Verification items for the finished model (mm, model axes). Face numbers are marked on the shaded views. A direction names the side the tool comes from. Give positions to 0.01 mm unless a question says otherwise; leave off trailing zeros. Write each loop counter-clockwise with the first axis right and the second up, starting at its lowest first coordinate (ties: lowest second). Pieces come first, ordered by that corner, then holes. Notation, with made-up numbers: (0, 18.5) - (13, 18.5) arc R34 ccw to (13, 54.5) - close; hole circle Ø2 at (22, -30.5). An arc over 180 degrees is marked (long way). Put each result on its own line as item: value.
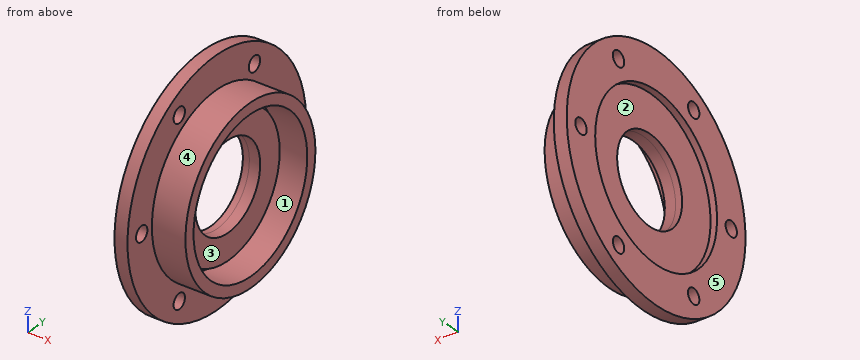
from build123d import *

# Parameters (mm, degrees)
SKETCH2_R           = 7
CUT_EXTRUDE1_DEPTH  = 12
SKETCH3_R           = 40
CUT_EXTRUDE2_DEPTH  = 6
SKETCH4_R           = 64
SKETCH4_R_2         = 40
BOSS_EXTRUDE1_DEPTH = 10


with BuildPart() as part:
    # Sketch1 → Revolve1 (revolve)
    with BuildSketch(Plane.XY, mode=Mode.PRIVATE) as revolve1_sk:
        Polygon((0, 75), (0, 110), (12, 110), (12, 80), (43, 80), (43, 70), (12, 70), (12, 0), (6, 0), (6, 75), align=None)
    revolve(revolve1_sk.sketch.rotate(Axis((0, 0, 0), (1, 0, 0)), 90), axis=Axis((0, 0, 0), (1, 0, 0)))

    # Sketch2 → Cut-Extrude1 (cut)
    with BuildSketch(Plane.ZY):
        with Locations((0, 92.5)):
            Circle(SKETCH2_R)
        with Locations((80.10734985, 46.25)):
            Circle(SKETCH2_R)
        with Locations((80.10734985, -46.25)):
            Circle(SKETCH2_R)
        with Locations((0, -92.5)):
            Circle(SKETCH2_R)
        with Locations((-80.10734985, -46.25)):
            Circle(SKETCH2_R)
        with Locations((-80.10734985, 46.25)):
            Circle(SKETCH2_R)
    extrude(amount=-CUT_EXTRUDE1_DEPTH, mode=Mode.SUBTRACT)

    # Sketch3 → Cut-Extrude2 (cut)
    with BuildSketch(Plane.ZY.offset(-6)):
        Circle(SKETCH3_R)
    extrude(amount=-CUT_EXTRUDE2_DEPTH, mode=Mode.SUBTRACT)

    # Sketch4 → Boss-Extrude1 (add)
    with BuildSketch(Plane(origin=(12, 0, 0), x_dir=(0, 0, -1), z_dir=(1, 0, 0))):
        with Locations(Location((0, 0, 0), (0, 0, 180))):
            Circle(SKETCH4_R)
        with Locations(Location((0, 0, 0), (0, 0, 180))):
            Circle(SKETCH4_R_2, mode=Mode.SUBTRACT)
    extrude(amount=BOSS_EXTRUDE1_DEPTH)


solid = part.part
Q1. Set-up check for the marked faces 1 and 2: record each of +Z, -Z, +X, -X, +Y, -Y from which the full face is reachable in a straight line by a thin tool's end or side.
Answers follow:
face 1: +X
face 2: -X
Q2. Section check A-A, the plane z = 0. Give the number of separate pieces and of enclosed holes in the cut face, plus the area to 3 significant figures.
Answers follow:
separate pieces: 4
enclosed holes: 0
area: 2,020 mm2
Q3. Section check C-C, the plane x = 18.5. Record the cut outline in (y, z).
Answers follow:
outline: circle Ø160 at (0, 0); circle Ø128 at (0, 0); hole circle Ø140 at (0, 0); hole circle Ø80 at (0, 0)
Q4. Section check D-D, the plane z = 27. Record the cut outline in (x, y), plus the area to 3 significant figures.
Answers follow:
outline: (0, -106.63) - (12, -106.63) - (12, -75.31) - (43, -75.31) - (43, -64.58) - (12, -64.58) - (12, -58.03) - (22, -58.03) - (22, -29.51) - (6, -29.51) - (6, -69.97) - (0, -69.97) - close; (0, 69.97) - (6, 69.97) - (6, 29.51) - (22, 29.51) - (22, 58.03) - (12, 58.03) - (12, 64.58) - (43, 64.58) - (43, 75.31) - (12, 75.31) - (12, 106.63) - (0, 106.63) - close
area: 2,600 mm2
Q5. Go/stop test with flat-tipped pins: pin 1 Ø18 at (y, z) = (46.25, 80.11) entering from +X; pin 2 Ø1.5 at (x, y) = (10.5, 24) entering from +Z; pin 3 Ø3 at (x, y) = (4.5, -5.5) entering from -Z. Record where each tip stops, or that it passes through.
Answers follow:
pin 1: stops at x = 12
pin 2: stops at z = 107.51
pin 3: stops at z = -109.93
Q6. Scan lines: line 1 along Z through (x, y) = (18.5, 45); line 2 along Z through (x, y) = (9, -46); line 3 along Z through (x, y) = (5, 46). Record each from-to range of solid material in increasing order.
Answers follow:
line 1: z = -66.14 to -53.62, -45.51 to 45.51, 53.62 to 66.14
line 2: z = -99.92 to -87.1, -73.11 to 73.11, 87.1 to 99.92
line 3: z = -99.92 to -87.1, -73.11 to -59.24, 59.24 to 73.11, 87.1 to 99.92
Q7. Release check for a two-part mould opening along Z. For the marked faces 3, 4 and 5 record: released by +Z, released by -Z, zero draft, split by the parting line, or undercut.
Answers follow:
face 3: undercut
face 4: split by the parting line
face 5: zero draft
Q8. Section check B-B, the plane y = 0. Record the cut outline in (x, z).
Answers follow:
outline: (0, -110) - (12, -110) - (12, -80) - (43, -80) - (43, -70) - (12, -70) - (12, -64) - (22, -64) - (22, -40) - (6, -40) - (6, -75) - (0, -75) - close; (0, 75) - (6, 75) - (6, 40) - (22, 40) - (22, 64) - (12, 64) - (12, 70) - (43, 70) - (43, 80) - (12, 80) - (12, 110) - (0, 110) - close
